Check sheet for the modelled part. Datum: model origin and axes. Units: mm. Face numbers are marked on the shaded views. A direction names the side the tool comes from. Coordinates: 2 decimals unless noted, no trailing zeros. Write each loop counter-clockwise with the first axis right and the second up, starting at its lowest first coordinate (ties: lowest second). Pieces come first, ordered by that corner, then holes. Notation, with made-up numbers: (55.5, 37) - (74.5, 37) arc R13 cw to (74.5, 42) - close; hole circle Ø9 at (-22.5, 84). An arc over 180 degrees is marked (long way). Use one line per item in the form item = value. Start each with the question number.
1. Cross-section at D-D on y = -38.1. Give the number of separate pieces and of enclosed holes in the cut face, then the cut area to 3 significant figures.
2. Cross-section at C-C on z = 577. Record the boundary of the cut face in (x, y), then the cut area to 3 significant figures.
3. Tool access check on the marked faces 5 and 6. Record the directions out of +Z, -Z, +X, -X, +Y, -Y that give a thin tool (end or side, any length) a straight path to the whole face; none if there is none.
4. Go/stop test with flat-tipped pins: pin 1 Ø6 at (y, z) = (24, 248) entering from -X; pin 2 Ø23 at (x, y) = (1200, -37.5) entering from -Z; pin 3 Ø12.5 at (y, z) = (-56, 33.5) entering from -X; pin 4 Ø23 at (x, y) = (1174.5, -48) entering from +Z. Record where each tip stops, or that it passes through.
5. Draft check along X on the marked faces 1, 2, 3 and 4. Enter one of: +X half, -X half, draft (parallel to the pull), parting line (faces both ways), or undercut.
6. Scan lines: line 1 along Y through (x, z) = (88.9, 118); line 2 along Z through (x, y) = (1083, 1); line 3 along X through (y, z) = (111, 170). Record each from-to range of solid material in increasing order.
7. Cross-section at B-B on y = 182. Record the boundary of the cut face in (x, z), then the cut area to 3 significant figures.
8. Cross-section at A-A on x = 533. Record the boundary of the cut face in (y, z), then the cut area to 3 significant figures.
```python
from build123d import *

# Parameters (mm, degrees)
SKETCH1_W           = 1270
SKETCH1_H           = 1219.2
BOSS_EXTRUDE1_DEPTH = 203.2
SKETCH2_W           = 965.2
SKETCH2_H           = 914.4
CUT_EXTRUDE2_DEPTH  = 203.2
SKETCH4_W           = 25.4
SKETCH4_H           = 76.2
SKETCH4_W_2         = 76.2
SKETCH4_H_2         = 25.4
BOSS_EXTRUDE2_DEPTH = 76.2
SKETCH6_R           = 25.4
CUT_EXTRUDE3_DEPTH  = 127
SKETCH7_R           = 25.4
CUT_EXTRUDE4_DEPTH  = 127
SKETCH8_R           = 25.4
CUT_EXTRUDE5_DEPTH  = 127
SKETCH9_R           = 25.4
CUT_EXTRUDE6_DEPTH  = 127
BOSS_EXTRUDE3_DEPTH = 127
SKETCH11_R          = 25.4
BOSS_EXTRUDE4_DEPTH = 508
BOSS_EXTRUDE5_START = 508
SKETCH12_R          = 25.4
BOSS_EXTRUDE5_DEPTH = 508


with BuildPart() as part:
    # Sketch1 → Boss-Extrude1 (new body)
    with BuildSketch(Plane(origin=(0, 0, 0), x_dir=(1, 0, 0), z_dir=(0, 1, 0))):
        with Locations((635, -609.6)):
            Rectangle(SKETCH1_W, SKETCH1_H)
    extrude(amount=BOSS_EXTRUDE1_DEPTH)

    # Sketch2 → Cut-Extrude2 (cut)
    with BuildSketch(Plane(origin=(0, 203.2, 0), x_dir=(1, 0, 0), z_dir=(0, 1, 0))):
        with Locations((635, -609.6)):
            Rectangle(SKETCH2_W, SKETCH2_H)
    extrude(amount=-CUT_EXTRUDE2_DEPTH, mode=Mode.SUBTRACT)

    # Sketch4 → Boss-Extrude2 (add)
    with BuildSketch(Plane(origin=(0, 0, 0), x_dir=(-1, 0, 0), z_dir=(0, -1, 0))):
        with Locations((-38.1, -1130.3)):
            Rectangle(SKETCH4_W, SKETCH4_H)
        with Locations((-114.3, -1130.3)):
            Rectangle(SKETCH4_W, SKETCH4_H)
        with Locations((-1181.1, -1181.1)):
            Rectangle(SKETCH4_W_2, SKETCH4_H_2)
        with Locations((-1181.1, -1104.9)):
            Rectangle(SKETCH4_W_2, SKETCH4_H_2)
        with Locations((-1231.9, -88.9)):
            Rectangle(SKETCH4_W, SKETCH4_H)
        with Locations((-1155.7, -88.9)):
            Rectangle(SKETCH4_W, SKETCH4_H)
        with Locations((-88.9, -114.3)):
            Rectangle(SKETCH4_W_2, SKETCH4_H_2)
        with Locations((-88.9, -38.1)):
            Rectangle(SKETCH4_W_2, SKETCH4_H_2)
    extrude(amount=BOSS_EXTRUDE2_DEPTH)

    # Sketch6 → Cut-Extrude3 (cut)
    with BuildSketch(Plane.ZY.offset(-25.4)):
        with Locations((1130.3, -38.1)):
            Circle(SKETCH6_R)
    extrude(amount=-CUT_EXTRUDE3_DEPTH, mode=Mode.SUBTRACT)

    # Sketch7 → Cut-Extrude4 (cut)
    with BuildSketch(Plane.XY.offset(1193.8)):
        with Locations((1181.1, -38.1)):
            Circle(SKETCH7_R)
    extrude(amount=-CUT_EXTRUDE4_DEPTH, mode=Mode.SUBTRACT)

    # Sketch8 → Cut-Extrude5 (cut)
    with BuildSketch(Plane(origin=(1244.6, 0, 0), x_dir=(0, 0, -1), z_dir=(1, 0, 0))):
        with Locations((-88.9, -38.1)):
            Circle(SKETCH8_R)
    extrude(amount=-CUT_EXTRUDE5_DEPTH, mode=Mode.SUBTRACT)

    # Sketch9 → Cut-Extrude6 (cut)
    with BuildSketch(Plane(origin=(0, 0, 25.4), x_dir=(-1, 0, 0), z_dir=(0, 0, -1))):
        with Locations((-88.9, -38.1)):
            Circle(SKETCH9_R)
    extrude(amount=-CUT_EXTRUDE6_DEPTH, mode=Mode.SUBTRACT)

    # Sketch10 → Boss-Extrude3 (add)
    with BuildSketch(Plane(origin=(0, 0, 0), x_dir=(-1, 0, 0), z_dir=(0, 0, -1))):
        Polygon((-584.2, 152.4), (-635, 152.4), (-685.8, 152.4), (-685.8, 50.8), (-584.2, 50.8), align=None)
    extrude(amount=BOSS_EXTRUDE3_DEPTH)

    # Sketch11 → Boss-Extrude4 (add)
    with BuildSketch(Plane.ZY.offset(-584.2)):
        with Locations((-63.5, 101.6)):
            Circle(SKETCH11_R)
    extrude(amount=BOSS_EXTRUDE4_DEPTH)

    # Sketch12 → Boss-Extrude5 (add)
    with BuildSketch(Plane(origin=(685.8, 0, 0), x_dir=(0, 0, -1), z_dir=(1, 0, 0)).offset(BOSS_EXTRUDE5_START)):
        with Locations(Location((63.5, 101.6, 0), (0, 0, 180))):
            Circle(SKETCH12_R)
    extrude(amount=-BOSS_EXTRUDE5_DEPTH)


solid = part.part
```
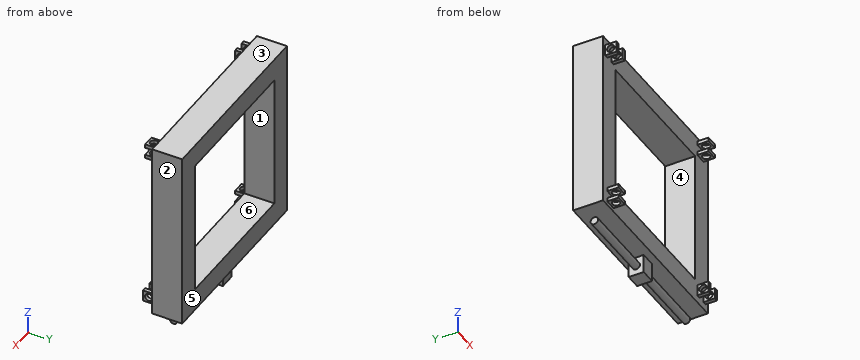
Final values:
q1.separate_pieces = 16
q1.enclosed_holes = 0
q1.area = 5,160 mm²
q2.outline = (0, 0) - (152.4, 0) - (152.4, 203.2) - (0, 203.2) - close; (1117.6, 0) - (1270, 0) - (1270, 203.2) - (1117.6, 203.2) - close
q2.area = 61,900 mm²
q3.face_5 = +Z, -Z, +X, -X, +Y
q3.face_6 = +Y, -Y
q4.pin_1 = 0
q4.pin_2 = 1092.2
q4.pin_3 = 50.8
q4.pin_4 = 127
q5.face_1 = undercut
q5.face_2 = +X half
q5.face_3 = draft
q5.face_4 = undercut
q6.line_1 = -76.2 to -63.5, -12.7 to 203.2
q6.line_2 = 0 to 152.4, 1066.8 to 1219.2
q6.line_3 = 0 to 152.4, 1117.6 to 1270
q7.outline = (0, 0) - (1270, 0) - (1270, 1219.2) - (0, 1219.2) - close; hole (152.4, 152.4) - (1117.6, 152.4) - (1117.6, 1066.8) - (152.4, 1066.8) - close
q7.area = 666,000 mm²
q8.outline = (0, 0) - (203.2, 0) - (203.2, 152.4) - (0, 152.4) - close; (0, 1066.8) - (203.2, 1066.8) - (203.2, 1219.2) - (0, 1219.2) - close; circle Ø50.8 at (101.6, -63.5)
q8.area = 64,000 mm²
